from build123d import *

# Parameters (mm, degrees)
BOSS_EXTRUDE1_DEPTH = 12.7
BOSS_EXTRUDE2_DEPTH = 25.4
SKETCH4_W           = 8.89
SKETCH4_H           = 6.35
BOSS_EXTRUDE3_DEPTH = 25.4
SKETCH5_R           = 2.54
CUT_EXTRUDE1_DEPTH  = 7.35
SKETCH6_W           = 20.066
SKETCH6_H           = 42.4
SKETCH6_R           = 2.25
BOSS_EXTRUDE4_DEPTH = 12.7
SKETCH7_R           = 6.35
SKETCH7_R_2         = 2.25
CUT_EXTRUDE2_DEPTH  = 6.35
SKETCH8_W           = 19.05
SKETCH8_H           = 42.4
CUT_EXTRUDE3_DEPTH  = 6.35
FILLET1_R           = 6.35
FILLET2_R           = 3.175


with BuildPart() as part:
    # Sketch1 → Boss-Extrude1 (new body)
    with BuildSketch(Plane.XY):
        Polygon((3833.667818581, -3.138), (3791.065892699, -3.138), (3781.25185564, -8.5), (3843.48185564, -8.5), align=None)
        with BuildLine():
            Line((3825.67435564, 0), (3799.05935564, 0))
            ThreePointArc((3799.05935564, 0), (3797.366063058, -2.180040562), (3794.834842884, -1.078795335))
            Line((3794.834842884, -1.078795335), (3791.065892699, -3.138))
            Line((3791.065892699, -3.138), (3833.667818581, -3.138))
            Line((3833.667818581, -3.138), (3829.898868396, -1.078795335))
            ThreePointArc((3829.898868396, -1.078795335), (3827.367648222, -2.180040562), (3825.67435564, 0))
        make_face()
        with BuildLine():
            Line((3843.48185564, -3.138), (3843.48185564, 0))
            Line((3843.48185564, 0), (3830.17435564, 0))
            ThreePointArc((3830.17435564, 0), (3830.104396202, -0.556707418), (3829.898868396, -1.078795335))
            Line((3829.898868396, -1.078795335), (3833.667818581, -3.138))
            Line((3833.667818581, -3.138), (3843.48185564, -3.138))
        make_face()
        Polygon((3812.36685564, 8.5), (3822.180892699, 3.138), (3843.48185564, 3.138), (3843.48185564, 8.5), align=None)
        with BuildLine():
            Line((3843.48185564, 3.138), (3822.180892699, 3.138))
            Line((3822.180892699, 3.138), (3825.949842884, 1.078795335))
            ThreePointArc((3825.949842884, 1.078795335), (3828.481063058, 2.180040562), (3830.17435564, 0))
            Line((3830.17435564, 0), (3843.48185564, 0))
            Line((3843.48185564, 0), (3843.48185564, 3.138))
        make_face()
        with BuildLine():
            Line((3822.180892699, 3.138), (3802.552818581, 3.138))
            Line((3802.552818581, 3.138), (3798.783868396, 1.078795335))
            ThreePointArc((3798.783868396, 1.078795335), (3798.989396202, 0.556707418), (3799.05935564, 0))
            Line((3799.05935564, 0), (3825.67435564, 0))
            ThreePointArc((3825.67435564, 0), (3825.744315078, 0.556707418), (3825.949842884, 1.078795335))
            Line((3825.949842884, 1.078795335), (3822.180892699, 3.138))
        make_face()
        Polygon((3812.36685564, 8.5), (3802.552818581, 3.138), (3822.180892699, 3.138), align=None)
        Polygon((3781.25185564, 8.5), (3781.25185564, 3.138), (3802.552818581, 3.138), (3812.36685564, 8.5), align=None)
        with BuildLine():
            Line((3802.552818581, 3.138), (3781.25185564, 3.138))
            Line((3781.25185564, 3.138), (3781.25185564, 0))
            Line((3781.25185564, 0), (3794.55935564, 0))
            ThreePointArc((3794.55935564, 0), (3796.252648222, 2.180040562), (3798.783868396, 1.078795335))
            Line((3798.783868396, 1.078795335), (3802.552818581, 3.138))
        make_face()
        with BuildLine():
            Line((3794.55935564, 0), (3781.25185564, 0))
            Line((3781.25185564, 0), (3781.25185564, -3.138))
            Line((3781.25185564, -3.138), (3791.065892699, -3.138))
            Line((3791.065892699, -3.138), (3794.834842884, -1.078795335))
            ThreePointArc((3794.834842884, -1.078795335), (3794.629315078, -0.556707418), (3794.55935564, 0))
        make_face()
        Polygon((3791.065892699, -3.138), (3781.25185564, -3.138), (3781.25185564, -8.5), align=None)
        Polygon((3843.48185564, -3.138), (3833.667818581, -3.138), (3843.48185564, -8.5), align=None)
    extrude(amount=BOSS_EXTRUDE1_DEPTH)

    # Sketch3 → Boss-Extrude2 (add)
    with BuildSketch(Plane(origin=(0, 8.5, 0), x_dir=(1, 0, 0), z_dir=(0, 1, 0))):
        Polygon((3831.44225564, 0), (3831.44225564, -6.35), (3840.33225564, -6.35), (3840.33225564, -12.7), (3843.48185564, -12.7), (3843.48185564, 0), align=None)
    extrude(amount=BOSS_EXTRUDE2_DEPTH)

    # Sketch4 → Boss-Extrude3 (add)
    with BuildSketch(Plane(origin=(0, 8.5, 0), x_dir=(1, 0, 0), z_dir=(0, 1, 0))):
        with Locations((3785.69685564, -3.175)):
            Rectangle(SKETCH4_W, SKETCH4_H)
    extrude(amount=BOSS_EXTRUDE3_DEPTH)

    # Sketch5 → Cut-Extrude1 (cut, through all)
    with BuildSketch(Plane.XY.offset(6.35)):
        with Locations((3835.76025564, 27.55)):
            Circle(SKETCH5_R)
        with Locations((3835.76025564, 17.644)):
            Circle(SKETCH5_R)
        with Locations((3786.23025564, 17.644)):
            Circle(SKETCH5_R)
        with Locations((3786.23025564, 27.55)):
            Circle(SKETCH5_R)
    extrude(amount=-CUT_EXTRUDE1_DEPTH, mode=Mode.SUBTRACT)

    # Sketch6 → Boss-Extrude4 (add)
    with BuildSketch(Plane(origin=(0, 0, 0), x_dir=(-1, 0, 0), z_dir=(0, 0, -1))):
        with Locations((-3853.51485564, 12.7)):
            Rectangle(SKETCH6_W, SKETCH6_H)
        with Locations((-3853.51485564, 0)):
            Circle(SKETCH6_R, mode=Mode.SUBTRACT)
        with Locations((-3853.51485564, 23.4830509)):
            Circle(SKETCH6_R, mode=Mode.SUBTRACT)
    extrude(amount=-BOSS_EXTRUDE4_DEPTH)

    # Sketch7 → Cut-Extrude2 (cut)
    with BuildSketch(Plane(origin=(0, 0, 0), x_dir=(-1, 0, 0), z_dir=(0, 0, -1))):
        with Locations((-3827.92435564, 0)):
            Circle(SKETCH7_R)
        with Locations((-3827.92435564, 0)):
            Circle(SKETCH7_R_2, mode=Mode.SUBTRACT)
        with Locations((-3796.80935564, 0)):
            Circle(SKETCH7_R)
        with Locations((-3796.80935564, 0)):
            Circle(SKETCH7_R_2, mode=Mode.SUBTRACT)
    extrude(amount=-CUT_EXTRUDE2_DEPTH, mode=Mode.SUBTRACT)

    # Sketch8 → Cut-Extrude3 (cut)
    with BuildSketch(Plane(origin=(0, 0, 0), x_dir=(-1, 0, 0), z_dir=(0, 0, -1))):
        with Locations((-3854.02285564, 12.7)):
            Rectangle(SKETCH8_W, SKETCH8_H)
    extrude(amount=-CUT_EXTRUDE3_DEPTH, mode=Mode.SUBTRACT)

    # Fillet1
    fillet1_edges = [part.edges().sort_by_distance(p)[0] for p in [
        (3844.49785564, -8.5, 3.175),
        (3781.25185564, -8.5, 6.35),
        (3863.54785564, 33.9, 9.525),
        (3863.54785564, -8.5, 9.525),
    ]]
    fillet(fillet1_edges, radius=FILLET1_R)

    # Fillet2
    fillet2_edges = [part.edges().sort_by_distance(p)[0] for p in [
        (3844.49785564, 33.9, 3.175),
        (3831.44225564, 33.9, 3.175),
        (3781.25185564, 33.9, 3.175),
        (3790.14185564, 33.9, 3.175),
    ]]
    fillet(fillet2_edges, radius=FILLET2_R)


solid = part.part
Check sheet for the modelled part. Datum: model origin and axes. Units: mm. A direction names the side the tool comes from. Give positions to 0.01 mm unless a question says otherwise; leave off trailing zeros. Write each loop counter-clockwise with the first axis right and the second up, starting at its lowest first coordinate (ties: lowest second). Pieces come first, ordered by that corner, then holes. Notation, with made-up numbers: (66.25, 71) -> (92.25, 71) arc R10 cw to (92.25, 77) -> close; hole circle Ø2 at (-15, 10.5). An arc over 180 degrees is marked (long way). Write item = value, one per line.
Item 1: Tool access check on faces 4 (the cylindrical face through (3834.27, 0.28, 3.13)), 5 (the cylindrical face through (3843.59, 32.95, 3.22)), 6 (the flat face through (3844.498, 14, 3)), 7 (the cylindrical face through (3842.59, -6.69, 3.22)), 8 (the flat face through (3790.142, 19, 3)). Record the directions out of +Z, -Z, +X, -X, +Y, -Y that give a thin tool (end or side, any length) a straight path to the whole face; none if there is none.
Output:
face_4 = -Z
face_5 = -Z, +X, +Y
face_6 = -Z, +X, +Y, -Y
face_7 = -Z, +X, -Y
face_8 = +Z, -Z, +Y
Item 2: Sectioned sample at D-D on y = 22.5. Record the boundary of the cut face in (x, z), and give its area (3 significant figures).
Output:
outline = (3781.25, 0) -> (3790.14, 0) -> (3790.14, 6.35) -> (3781.25, 6.35) -> close; (3831.44, 0) -> (3844.5, 0) -> (3844.5, 6.35) -> (3851.49, 6.35) -> (3851.49, 12.7) -> (3840.33, 12.7) -> (3840.33, 6.35) -> (3831.44, 6.35) -> close; (3855.54, 6.35) -> (3863.55, 6.35) -> (3863.55, 12.7) -> (3855.54, 12.7) -> close
area = 261 mm^2
Item 3: Sectioned sample at A-A on y = 12. Record the boundary of the cut face in (x, z), and give its area (3 significant figures).
Output:
outline = (3781.25, 0) -> (3790.14, 0) -> (3790.14, 6.35) -> (3781.25, 6.35) -> close; (3831.44, 0) -> (3844.5, 0) -> (3844.5, 6.35) -> (3863.55, 6.35) -> (3863.55, 12.7) -> (3840.33, 12.7) -> (3840.33, 6.35) -> (3831.44, 6.35) -> close
area = 287 mm^2
Item 4: Release check for a two-part mould opening along Y. For faces 1 (the cylindrical face through (3782.207, 32.995, 3.131)), 2 (the cylindrical face through (3788.577, 26.577, 3.219)), 3 (the cylindrical face through (3861.74, -6.59, 9.57)) record: +Y half, -Y half, draft (parallel to the pull), parting line (faces both ways), or undercut.
Output:
face_1 = +Y half
face_2 = undercut
face_3 = -Y half
Item 5: Sectioned sample at C-C on z = 5.5. Record the boundary of the cut face in (x, y) (3 decimals).
Output:
outline = (3781.252, -2.15) arc R6.35 ccw to (3787.602, -8.5) -> (3838.148, -8.5) arc R6.35 ccw to (3844.498, -2.15) -> (3844.498, 30.725) arc R3.175 ccw to (3841.323, 33.9) -> (3834.617, 33.9) arc R3.175 ccw to (3831.442, 30.725) -> (3831.442, 8.5) -> (3790.142, 8.5) -> (3790.142, 30.725) arc R3.175 ccw to (3786.967, 33.9) -> (3784.427, 33.9) arc R3.175 ccw to (3781.252, 30.725) -> close; hole circle Ø5.08 at (3786.23, 17.644); hole circle Ø5.08 at (3786.23, 27.55); hole circle Ø12.7 at (3796.809, 0); hole circle Ø12.7 at (3827.924, 0); hole circle Ø5.08 at (3835.76, 17.644); hole circle Ø5.08 at (3835.76, 27.55)
Item 6: Gauge pin test, flat ends, axial feed: pin 1 (7 mm diameter, centred on y = 20.5, z = 10.5, fed in from -X); pin 2 (1 mm diameter, centred on x = 3814.5, z = 10.5, fed in from +Y); pin 3 (4.5 mm diameter, centred on x = 3835.5, y = 24.5, fed in from +Z). Record the tip position at first contact, or that the pin passes through.
Output:
pin_1 = 3840.33
pin_2 = 8.5
pin_3 = 6.35
Item 7: Scan lines: probe 1 along X at (y, z) = (23, 4); probe 2 along X at (y, z) = (26.5, 2.5); probe 3 along X at (y, z) = (18.5, 9.5). Record each from-to range of solid material in increasing order. Write a range as from..to.
Output:
probe_1 = 3781.25..3790.14, 3831.44..3844.5
probe_2 = 3781.25..3783.92, 3788.54..3790.14, 3831.44..3833.45, 3838.07..3844.5
probe_3 = 3840.33..3863.55
Item 8: Sectioned sample at B-B on x = 3836. Record the boundary of the cut face in (y, z).
Output:
outline = (-8.5, 0) -> (15.12, 0) -> (15.12, 6.35) -> (8.5, 6.35) -> (8.5, 12.7) -> (-8.5, 12.7) -> close; (20.17, 0) -> (25.02, 0) -> (25.02, 6.35) -> (20.17, 6.35) -> close; (30.08, 0) -> (33.9, 0) -> (33.9, 6.35) -> (30.08, 6.35) -> close
